Check sheet for the modelled part. Datum: model origin and axes. Units: mm. A direction names the side the tool comes from. Round coordinates to 2 decimals unless told otherwise and drop trailing zeros. Write each loop counter-clockwise with the first axis right and the second up, starting at its lowest first coordinate (ties: lowest second). Pieces come first, ordered by that corner, then holes. Notation, with made-up numbers: (75, -24.75) -> (89, -24.75) arc R25 ccw to (89, 5.25) -> close; hole circle Ø4 at (56.25, 52). An arc over 180 degrees is marked (long way). Answer as a JSON object with one key per item and string values. Group by question number.
```python
from build123d import *

# Parameters (mm, degrees)
BASE_EXTRUSION_DEPTH    = 1.5
ESQUISSE2_R             = 1
ENL_V_MAT_EXTRU_1_DEPTH = 2.5
ESQUISSE3_R             = 1
BOSS_EXTRU_1_DEPTH      = 5.5
ESQUISSE4_R             = 6
BOSS_EXTRU_2_DEPTH      = 0.5
ESQUISSE5_R             = 4.5
ENL_V_MAT_EXTRU_2_DEPTH = 8.5


with BuildPart() as part:
    # Esquisse1 → Base-Extrusion (new body)
    with BuildSketch(Plane.XY):
        with BuildLine():
            ThreePointArc((12.328808061, -5.500044708), (11.691342951, 6.75), (1.401225592, 13.427083333))
            ThreePointArc((1.401225592, 13.427083333), (0, 14), (-1.401225592, 13.427083333))
            ThreePointArc((-1.401225592, 13.427083333), (-11.691342951, 6.75), (-12.328808061, -5.500044708))
            ThreePointArc((-12.328808061, -5.500044708), (-12.124355653, -7), (-10.927582469, -7.927038626))
            ThreePointArc((-10.927582469, -7.927038626), (0, -13.5), (10.927582469, -7.927038626))
            ThreePointArc((10.927582469, -7.927038626), (12.124355653, -7), (12.328808061, -5.500044708))
        make_face()
    extrude(amount=BASE_EXTRUSION_DEPTH)

    # Esquisse2 → Enlèv. mat.-Extru.1 (cut, through all)
    with BuildSketch(Plane.XY.offset(1.5)):
        with Locations((0, 12)):
            Circle(ESQUISSE2_R)
        with Locations((10.392304845, -6)):
            Circle(ESQUISSE2_R)
        with Locations((-10.392304845, -6)):
            Circle(ESQUISSE2_R)
    extrude(amount=-ENL_V_MAT_EXTRU_1_DEPTH, mode=Mode.SUBTRACT)

    # Esquisse3 → Boss.-Extru.1 (add)
    with BuildSketch(Plane.XY.offset(1.5)):
        with Locations((10.392304845, 6)):
            Circle(ESQUISSE3_R)
        with Locations((0, -12)):
            Circle(ESQUISSE3_R)
        with Locations((-10.392304845, 6)):
            Circle(ESQUISSE3_R)
    extrude(amount=BOSS_EXTRU_1_DEPTH)

    # Esquisse4 → Boss.-Extru.2 (add)
    with BuildSketch(Plane(origin=(0, 0, 0), x_dir=(-1, 0, 0), z_dir=(0, 0, -1))):
        Circle(ESQUISSE4_R)
    extrude(amount=BOSS_EXTRU_2_DEPTH)

    # Esquisse5 → Enlèv. mat.-Extru.2 (cut, through all)
    with BuildSketch(Plane(origin=(0, 0, -0.5), x_dir=(-1, 0, 0), z_dir=(0, 0, -1))):
        Circle(ESQUISSE5_R)
    extrude(amount=-ENL_V_MAT_EXTRU_2_DEPTH, mode=Mode.SUBTRACT)


solid = part.part
```
(1) Scan lines: line 1 along Y through (x, z) = (0, 0.3); line 2 along Y through (x, z) = (-10.5, 4.75); line 3 along X through (y, z) = (-5.25, 1). Record each from-to range of solid material in increasing order.
(2) Access from +Z, -Z, +X, -X, +Y, -Y to the whole of each face (thin tool, end or side, straight path). Record for faces 4 (the cylindrical face through (-11.601, 6.904, 0.74)), 5 (the flat face through (-6.2, 0.4, 0)), 6 (the cylindrical face through (10.93, 6.843, 4.212)).
(3) Release check for a two-part mould opening along Y. For faces 1 (the cylindrical face through (-12.135, -6.981, 0.74)), 2 (the cylindrical face through (-11.129, 6.676, 4.212)), 3 (the flat face through (10, 6, 7)) record: pulls with the +Y half, pulls with the -Y half, needs draft (parallel to the pull), parting line crosses it, or undercut.
(4) Section check D-D on y = -12. Record the cut outline in (x, z).
(5) Go/stop test with flat-tipped pins: pin 1 Ø3 at (x, y) = (0, 12) entering from +Z; pin 2 Ø5 at (x, y) = (-10, 10.5) entering from -Z; pin 3 Ø1.8 at (x, y) = (-10.39, -6) entering from +Z; pin 4 Ø4 at (x, z) = (6.5, 1.5) entering from -Y. Record where each tip stops, or that it passes through.
(6) Section check C-C on z = 4. Record the cut outline in (x, y), then the cut area to 3 significant figures.
(7) Section check A-A on x = -10. Record the cut outline in (y, z), then the cut area to 3 significant figures.
(8) Section check B-B on y = 12. Record the cut outline in (x, z).
Data:
{
 "1": {"line 1": "y = -13.5 to -4.5, 4.5 to 11, 13 to 14", "line 2": "y = 5.01 to 6.99", "line 3": "x = -12.44 to -11.05, -9.73 to 9.73, 11.05 to 12.44"},
 "2": {"face 4": "+Z, -Z, -X", "face 5": "-Z", "face 6": "+Z"},
 "3": {"face 1": "undercut", "face 2": "parting line crosses it", "face 3": "needs draft"},
 "4": {"outline": "(-6.18, 0) -> (6.18, 0) -> (6.18, 1.5) -> (1, 1.5) -> (1, 7) -> (-1, 7) -> (-1, 1.5) -> (-6.18, 1.5) -> close"},
 "5": {"pin 1": "stops at z = 1.5", "pin 2": "stops at z = 0", "pin 3": "passes through", "pin 4": "stops at y = -12.73"},
 "6": {"outline": "circle Ø2 at (-10.39, 6); circle Ø2 at (0, -12); circle Ø2 at (10.39, 6)", "area": "9.42 mm²"},
 "7": {"outline": "(-9.07, 0) -> (-6.92, 0) -> (-6.92, 1.5) -> (-9.07, 1.5) -> close; (-5.08, 0) -> (9.07, 0) -> (9.07, 1.5) -> (6.92, 1.5) -> (6.92, 7) -> (5.08, 7) -> (5.08, 1.5) -> (-5.08, 1.5) -> close", "area": "34.6 mm²"},
 "8": {"outline": "(-6.18, 0) -> (-1, 0) -> (-1, 1.5) -> (-6.18, 1.5) -> close; (1, 0) -> (6.18, 0) -> (6.18, 1.5) -> (1, 1.5) -> close"}
}
